For this review, use the dimensioned drawing (mm, ordinates from the lowest corner) and the shaded views. Round coordinates to 2 decimals unless told otherwise and drop trailing zeros. Order: outer loops, then holes, each group sorted by start corner. A loop starts at its lowest first (then second) coordinate and runs counter-clockwise, first axis right, second up. Notation, with made-up numbers: (-14, 87) - (-2, 87) arc R31 cw to (-2, 113) - close; hole circle Ø1 at (-26.5, 1). An arc over 180 degrees is marked (long way). Write item = value, one per line.
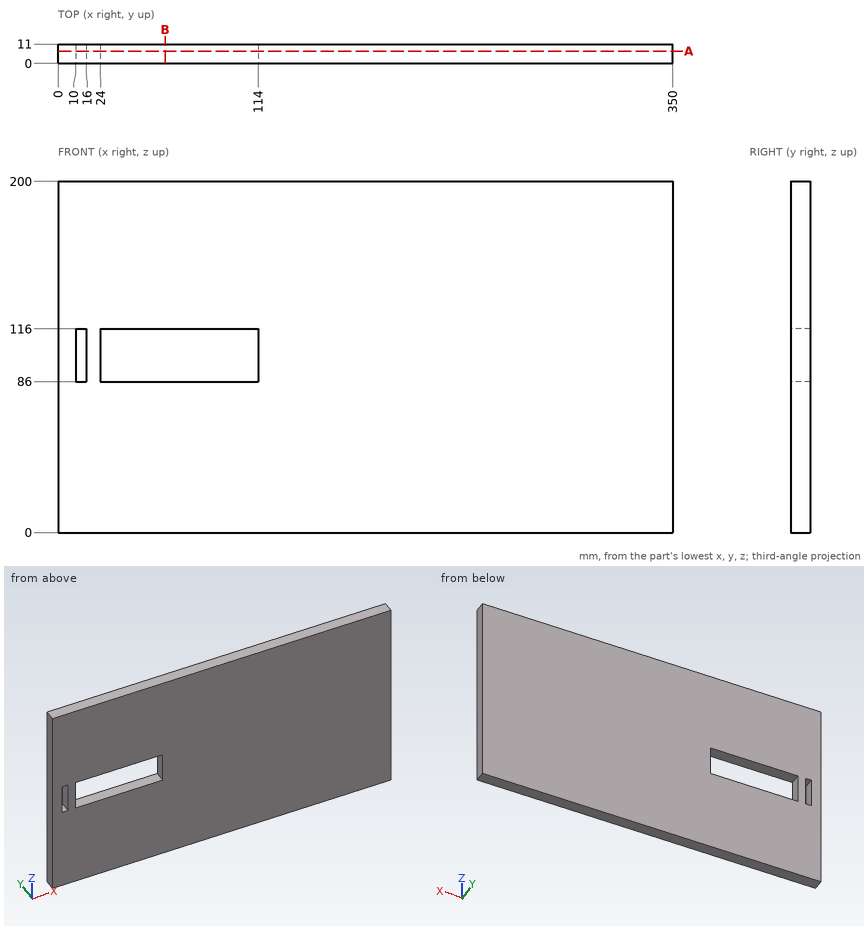
Item 1: For line 1 along X through (y, z) = (1.5, 110.5); line 2 along Z through (x, y) = (66, 0.75), list the stretches that pass through material, from the lowest coordinate up. Write a range as [from, to].
Data:
line_1 = [0, 10], [16, 24], [114, 350]
line_2 = [0, 86], [116, 200]
Item 2: Take a section at B-B, the plane x = 61. State the section outline as (y, z) points.
Data:
outline = (0, 0) - (11, 0) - (11, 86) - (0, 86) - close; (0, 116) - (11, 116) - (11, 200) - (0, 200) - close
Item 3: Take a section at A-A, the plane y = 7. State the section outline as (x, z) points, and give its area (3 significant figures).
Data:
outline = (0, 0) - (350, 0) - (350, 200) - (0, 200) - close; hole (10, 86) - (16, 86) - (16, 116) - (10, 116) - close; hole (24, 86) - (114, 86) - (114, 116) - (24, 116) - close
area = 67,100 mm2
